Geometry: final body of the model. Coordinates: model frame, mm. A direction names the side the tool comes from. Give positions to 0.01 mm unless a question says otherwise; leave off trailing zeros. Order: outer loops, then holes, each group sorted by start corner. A loop starts at its lowest first (then second) coordinate and runs counter-clockwise, first axis right, second up. Notation, with made-up numbers: (-22.5, -12) -> (1.5, -12) arc R33 cw to (1.5, 17) -> close; hole circle Ø9 at (54, -24). An arc over 180 degrees is marked (long way). One line per question, with ' | ' between items. Start each with the question number.
(1) First-contact query: pin 1 Ø3 at (x, y) = (-10, -13) entering from +Z; pin 2 Ø6 at (y, z) = (9, 6.5) entering from -X; pin 3 Ø6 at (x, z) = (-9.5, 8) entering from -Y. Flat tips, straight axial feed; report the tip coordinate or a pass-through.
(2) Section C-C (y = 14). Return loops of the section in (x, z), then the cut area to 3 significant figures.
(3) Section A-A (x = 0). Return loops of the section in (y, z).
(4) Set-up query: faces 4 (the face through (-2.38, -10.74, 6.45)), 5 (the face through (16.07, 16, 1.48)). Return all of +Z, -Z, +X, -X, +Y, -Y with unobstructed straight access to the full face (end or side cutting, diameter ignored); none if empty.
(5) Section D-D (z = 2). Return loops of the section in (x, y) (3 decimals), then the cut area to 3 significant figures.
(6) Ray query, L1, parallel to Y at x = 0, z = 7; L2, parallel to Z at x = -14, y = -6.5; L3, parallel to X at y = 11.5, z = 2.5. Return the intervals inside material, ascending.
(7) Mould query, pull axis X, two halves, no side actions, for faces 1 (the face through (17.5, 0, 1)), 2 (the face through (-17.5, 0, 1)), 3 (the face through (7.2, 0.2, 3)). Classes: +X half, -X half, draft (parallel to the pull), parting line (faces both ways), or undercut.
```python
from build123d import *

# Parameters (mm, degrees)
F0_R     = 3.175
F0_R_2   = 13
F1_DEPTH = 3
F0_R_3   = 11
F0_R_4   = 7
F2_DEPTH = 10


with BuildPart() as f1:
    # F0 (on Top) → F1 (new body)
    with BuildSketch(Plane.XY):
        with BuildLine():
            ThreePointArc((17.5, 12.5), (16.0355339059, 16.0355339059), (12.5, 17.5))
            Line((12.5, 17.5), (-12.5, 17.5))
            ThreePointArc((-12.5, 17.5), (-16.0355339059, 16.0355339059), (-17.5, 12.5))
            Line((-17.5, 12.5), (-17.5, -12.5))
            ThreePointArc((-17.5, -12.5), (-16.0355339059, -16.0355339059), (-12.5, -17.5))
            Line((-12.5, -17.5), (12.5, -17.5))
            ThreePointArc((12.5, -17.5), (16.0355339059, -16.0355339059), (17.5, -12.5))
            Line((17.5, -12.5), (17.5, 12.5))
        make_face()
        with Locations((-12.325, -12.325)):
            Circle(F0_R, mode=Mode.SUBTRACT)
        with Locations((12.325, -12.325)):
            Circle(F0_R, mode=Mode.SUBTRACT)
        with Locations((-12.325, 12.325)):
            Circle(F0_R, mode=Mode.SUBTRACT)
        Circle(F0_R_2, mode=Mode.SUBTRACT)
        with Locations((12.325, 12.325)):
            Circle(F0_R, mode=Mode.SUBTRACT)
    extrude(amount=F1_DEPTH)



with BuildPart() as f1b:
    # F0 (on Top) → F1, piece 2 (new body)
    with BuildSketch(Plane.XY):
        Circle(F0_R_3)
        Circle(F0_R_4, mode=Mode.SUBTRACT)
    extrude(amount=F1_DEPTH)


with BuildPart() as f1_1:
    add(f1.part)

    add(f1b.part)  # F2 merges F1b
    # F0 (on Top) → F2 (join)
    with BuildSketch(Plane.XY):
        Circle(F0_R_2)
        Circle(F0_R_3, mode=Mode.SUBTRACT)
    extrude(amount=F2_DEPTH)


solid = f1_1.part
```
Response:
1) pin 1: stops at z = 3 | pin 2: stops at x = -11.53 | pin 3: stops at y = -11.26
2) outline: (-17.27, 0) -> (-15.02, 0) -> (-15.02, 3) -> (-17.27, 3) -> close; (-9.63, 0) -> (9.63, 0) -> (9.63, 3) -> (-9.63, 3) -> close; (15.02, 0) -> (17.27, 0) -> (17.27, 3) -> (15.02, 3) -> close | area: 71.3 mm^2
3) outline: (-17.5, 0) -> (-7, 0) -> (-7, 3) -> (-11, 3) -> (-11, 10) -> (-13, 10) -> (-13, 3) -> (-17.5, 3) -> close; (7, 0) -> (17.5, 0) -> (17.5, 3) -> (13, 3) -> (13, 10) -> (11, 10) -> (11, 3) -> (7, 3) -> close
4) face 4: +Z | face 5: +Z, -Z, +X, +Y
5) outline: (-17.5, -12.5) arc R5 ccw to (-12.5, -17.5) -> (12.5, -17.5) arc R5 ccw to (17.5, -12.5) -> (17.5, 12.5) arc R5 ccw to (12.5, 17.5) -> (-12.5, 17.5) arc R5 ccw to (-17.5, 12.5) -> close; hole circle Ø6.35 at (-12.325, -12.325); hole circle Ø6.35 at (-12.325, 12.325); hole circle Ø14 at (0, 0); hole circle Ø6.35 at (12.325, -12.325); hole circle Ø6.35 at (12.325, 12.325) | area: 923 mm^2
6) L1: y = -13 to -11, 11 to 13 | L2: z = 0 to 3 | L3: x = -17.5 to -15.39, -9.26 to 9.26, 15.39 to 17.5
7) face 1: +X half | face 2: -X half | face 3: undercut
